For this review, take the finished solid that the model builds, in its own axes (mm). A direction names the side the tool comes from. Coordinates: 2 decimals unless noted, no trailing zeros. Loops run counter-clockwise (first coordinate to the right, second up) from the corner with the lowest first, then second, coordinate; pieces in that order, holes last. Notation, with made-up numbers: M 21.5,18.25 L 68.5,18.25 A18 cw 68.5,39.25 Z; hole C 1.5,-22 d9. An arc over 180 degrees is marked long. Answer as a JSON object with one key per item and string values. Group by question number.
Item 1: Add section C-C (x = 2). State the section outline as (y, z) points.
Item 2: Wall thickness on L1, parallel to Z at x = 10.5, y = 4; L2, parallel to X at y = -2.5, z = 29.5; L3, parallel to Z at x = 18.5, y = 4: over which ranges is each line inside the solid? List them lowest first. Write a range as from..to.
Item 3: Tool access review of faces 4 (the face through (15.24, 0, 22)), 5 (the face through (-0.661, 5.037, 12.522)), 6 (the face through (-2, 0, 25.4)): name each direction out of +Z, -Z, +X, -X, +Y, -Y from which nothing blocks a thin tool from reaching the whole face with its end or side.
Item 4: Add section A-A (y = 0). State the section outline as (x, z) points, then the cut area to 3 significant figures.
Item 5: Insertion check: pin 1 (3 mm diameter, centred on x = 21, y = 0.5, fed in from -Z); pin 2 (2 mm diameter, centred on y = -2.5, z = 15.5, fed in from -X); pin 3 (1.5 mm diameter, centred on y = 0.5, z = 29, fed in from -X). Each pin has a flat end and moves straight along its axis. Give the tip position at first contact, or say it passes through.
Item 6: Mouldability with a two-part tool opening along X and no side actions: class faces 1 (the face through (0, 0, 28)), 2 (the face through (9, 0, 25.4)), 3 (the face through (20, 0, 19.05)) as +X half, -X half, draft (parallel to the pull), parting line (faces both ways), or undercut.
Item 7: Add section D-D (y = -2). State the section outline as (x, z) points.
Item 8: Add section B-B (z = 18.5). State the section outline as (x, y) points, then the cut area to 3 significant figures.
from build123d import *

# Parameters (mm, degrees)
F0_R     = 5.08
F1_DEPTH = 25.4
F2_W     = 25.4
F2_H     = 10.16
F3_DEPTH = 5.08
F4_W     = 10.16
F4_H     = 10.16
F5_DEPTH = 6.35


with BuildPart() as f1:
    # F0 (on Top) → F1 (new body)
    with BuildSketch(Plane.XY):
        Circle(F0_R)
    extrude(amount=F1_DEPTH)

    # F2 (on face) → F3 (join)
    with BuildSketch(Plane.XY.offset(25.4)):
        with Locations((12.7, 0)):
            Rectangle(F2_W, F2_H)
    extrude(amount=F3_DEPTH)

    # F4 (on face) → F5 (join)
    with BuildSketch(Plane(origin=(0, 0, 25.4), x_dir=(1, 0, 0), z_dir=(0, 0, -1))):
        with Locations((20.32, 0)):
            Rectangle(F4_W, F4_H)
    extrude(amount=F5_DEPTH)


solid = f1.part
From the geometry:
{
 "1": {"outline": "M -5.08,25.4 L -4.67,25.4 L -4.67,0 L 4.67,0 L 4.67,25.4 L 5.08,25.4 L 5.08,30.48 L -5.08,30.48 Z"},
 "2": {"L1": "z = 25.4..30.48", "L2": "x = 0..25.4", "L3": "z = 19.05..30.48"},
 "3": {"face 4": "-Z, +Y, -Y", "face 5": "-Z", "face 6": "+Z, -X, +Y, -Y"},
 "4": {"outline": "M -5.08,0 L 5.08,0 L 5.08,25.4 L 15.24,25.4 L 15.24,19.05 L 25.4,19.05 L 25.4,30.48 L 0,30.48 L 0,25.4 L -5.08,25.4 Z", "area": "452 mm²"},
 "5": {"pin 1": "stops at z = 19.05", "pin 2": "stops at x = -4.85", "pin 3": "stops at x = 0"},
 "6": {"face 1": "-X half", "face 2": "undercut", "face 3": "draft"},
 "7": {"outline": "M -4.67,0 L 4.67,0 L 4.67,25.4 L 15.24,25.4 L 15.24,19.05 L 25.4,19.05 L 25.4,30.48 L 0,30.48 L 0,25.4 L -4.67,25.4 Z"},
 "8": {"outline": "C 0,0 d10.16", "area": "81.1 mm²"}
}
